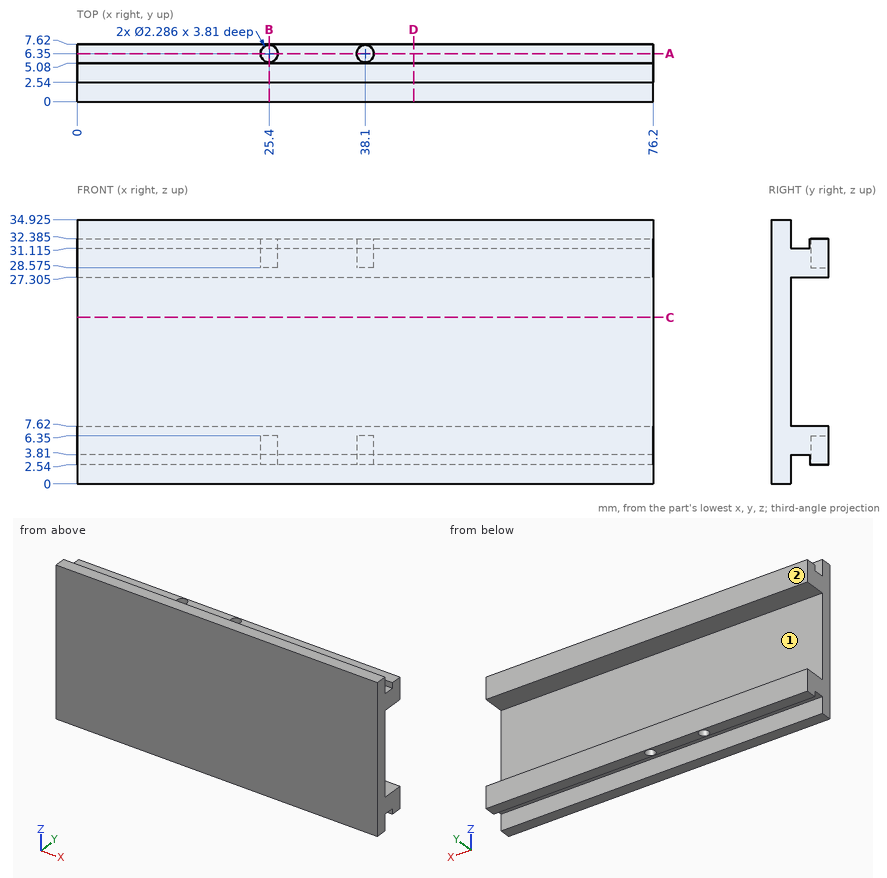
Input: dimensioned drawing with shaded views. Units: mm. Origin: part minimum x, y, z. Coordinates: 2 decimals unless noted, no trailing zeros. Write each loop counter-clockwise with the first axis right and the second up, starting at its lowest first coordinate (ties: lowest second). Pieces come first, ordered by that corner, then holes. Notation, with made-up numbers: (89.25, -6.5) -> (146.25, -6.5) arc R27 ccw to (146.25, 12.5) -> close; hole circle Ø5 at (2.25, 40). An arc over 180 degrees is marked (long way). Return JSON: item names as keys, results as strings. Group by question number.
1) Section query C-C, the plane z = 22. Return loops of the section in (x, y), plus the area to 3 significant figures.
2) Section query D-D, the plane x = 44.5. Return loops of the section in (y, z) (3 decimals), plus the area to 3 significant figures.
3) Section query A-A, the plane y = 6.35. Return loops of the section in (x, z) (3 decimals), plus the area to 3 significant figures.
4) Ray query, line 1 along X through (y, z) = (6.35, 5.1); line 2 along Z through (x, y) = (20, 4.75) (3 decimals); line 3 along Z through (x, y) = (46.5, 6.25) (3 decimals). Return the intervals inside material, ascending.
5) Contact query for flat-ended pins moving along their axis: P1, Ø3.5, axis at x = 38.1, y = 6.35, coming from the -Z side; P2, Ø1.3, axis at x = 32.5, y = 4, coming from the +Z side (3 decimals); P3, Ø1.1, axis at x = 38.5, y = 7, coming from the +Z side (3 decimals). Output: stop coordinate, or through.
6) Section query B-B, the plane x = 25.4. Return loops of the section in (y, z) (3 decimals), plus the area to 3 significant figures.
7) Mould query, pull axis Z, two halves, no side actions, for the marked faces 1 and 2. Classes: +Z half, -Z half, draft (parallel to the pull), parting line (faces both ways), or undercut.
From the geometry:
{
 "1": {"outline": "(0, 0) -> (76.2, 0) -> (76.2, 2.54) -> (0, 2.54) -> close", "area": "194 mm²"},
 "2": {"outline": "(0, 0) -> (2.54, 0) -> (2.54, 3.81) -> (5.08, 3.81) -> (5.08, 2.54) -> (7.62, 2.54) -> (7.62, 7.62) -> (2.54, 7.62) -> (2.54, 27.305) -> (7.62, 27.305) -> (7.62, 32.385) -> (5.08, 32.385) -> (5.08, 31.115) -> (2.54, 31.115) -> (2.54, 34.925) -> (0, 34.925) -> close", "area": "134 mm²"},
 "3": {"outline": "(0, 2.54) -> (24.257, 2.54) -> (24.257, 6.35) -> (26.543, 6.35) -> (26.543, 2.54) -> (36.957, 2.54) -> (36.957, 6.35) -> (39.243, 6.35) -> (39.243, 2.54) -> (76.2, 2.54) -> (76.2, 7.62) -> (0, 7.62) -> close; (0, 27.305) -> (76.2, 27.305) -> (76.2, 32.385) -> (39.243, 32.385) -> (39.243, 28.575) -> (36.957, 28.575) -> (36.957, 32.385) -> (26.543, 32.385) -> (26.543, 28.575) -> (24.257, 28.575) -> (24.257, 32.385) -> (0, 32.385) -> close", "area": "739 mm²"},
 "4": {"line 1": "0 to 24.26, 26.54 to 36.96, 39.24 to 76.2", "line 2": "3.81 to 7.62, 27.305 to 31.115", "line 3": "2.54 to 7.62, 27.305 to 32.385"},
 "5": {"P1": "z = 2.54", "P2": "z = 31.115", "P3": "z = 32.385"},
 "6": {"outline": "(0, 0) -> (2.54, 0) -> (2.54, 3.81) -> (5.08, 3.81) -> (5.08, 2.54) -> (5.207, 2.54) -> (5.207, 6.35) -> (7.493, 6.35) -> (7.493, 2.54) -> (7.62, 2.54) -> (7.62, 7.62) -> (2.54, 7.62) -> (2.54, 27.305) -> (7.62, 27.305) -> (7.62, 32.385) -> (7.493, 32.385) -> (7.493, 28.575) -> (5.207, 28.575) -> (5.207, 32.385) -> (5.08, 32.385) -> (5.08, 31.115) -> (2.54, 31.115) -> (2.54, 34.925) -> (0, 34.925) -> close", "area": "116 mm²"},
 "7": {"face 1": "undercut", "face 2": "draft"}
}
